Work out the finished part from the listing and answer in its coordinate system (mm). Face numbers are marked on the shaded views. A direction names the side the tool comes from. Give positions to 0.01 mm unless a question says otherwise; leave off trailing zeros. Order: outer loops, then holes, each group sorted by start corner. A loop starts at its lowest first (then second) coordinate and runs counter-clockwise, first axis right, second up. Notation, with made-up numbers: (-14, 17.5) - (30, 17.5) arc R31 ccw to (30, 45.5) - close; hole circle Ø8 at (30.5, 51.5). An arc over 180 degrees is marked (long way). Return JSON: item names as keys, results as strings. Group by question number.
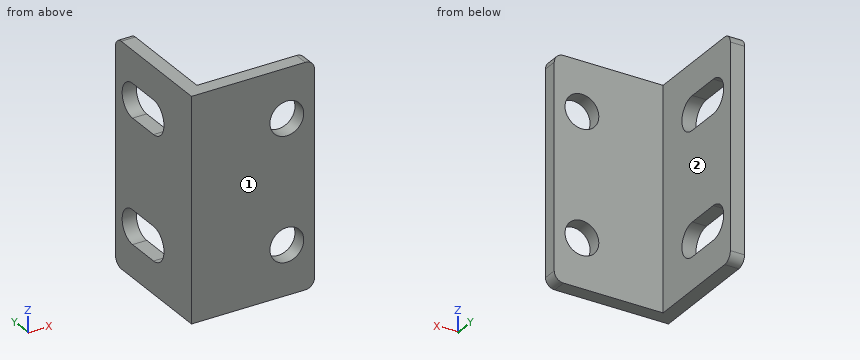
Autodesk Inventor part; units mm, degrees
ref_plane "to_cbm_1_1_XY" through (2.3, 15.5, -10) normal (1, 0, 0) x (0, 0, -1)
ref_plane "to_cbm_1_1_YZ" through (2.3, 15.5, -10) normal (0, 0, -1) x (0, 1, 0)
ref_plane "to_cbm_1_1_ZX" through (2.3, 15.5, -10) normal (0, 1, 0) x (1, 0, 0)
sketch "Sketch_2" plane through (0, 0, 0) normal (0, 1, 0) x (-1, 0, 0)
  line L0 (0, 18) -> (-18.5, 18)
  arc A0 (-18.5, 18) -> (-20, 16.5) centre (-18.5, 16.5) ccw
  line L1 (-20, 16.5) -> (-20, -16.5)
  arc A1 (-20, -16.5) -> (-18.5, -18) centre (-18.5, -16.5) ccw
  line L2 (-18.5, -18) -> (0, -18)
  line L3 (0, -18) -> (0, 18)
  circle A2 centre (-15.5, -10) radius 2.75
  circle A3 centre (-15.5, 10) radius 2.75
extrude "Extrusion1" add sketch "Sketch_2" along normal blind 2.3
sketch "Sketch_1" plane through (0, 0, 0) normal (1, 0, 0) x (0, 1, 0)
  line L0 (18.5, 18) -> (0, 18)
  line L1 (0, 18) -> (0, -18)
  line L2 (0, -18) -> (18.5, -18)
  arc A0 (18.5, -18) -> (20, -16.5) centre (18.5, -16.5) ccw
  line L3 (20, -16.5) -> (20, 16.5)
  arc A1 (20, 16.5) -> (18.5, 18) centre (18.5, 16.5) ccw
  line L4 (15.5, -7.25) -> (10, -7.25)
  arc A2 (10, -7.25) -> (10, -12.75) centre (10, -10) ccw
  line L5 (10, -12.75) -> (15.5, -12.75)
  arc A3 (15.5, -12.75) -> (15.5, -7.25) centre (15.5, -10) ccw
  line L6 (15.5, 12.75) -> (10, 12.75)
  arc A4 (10, 12.75) -> (10, 7.25) centre (10, 10) ccw
  line L7 (10, 7.25) -> (15.5, 7.25)
  arc A5 (15.5, 7.25) -> (15.5, 12.75) centre (15.5, 10) ccw
extrude "Extrusion2" add sketch "Sketch_1" along normal blind 2.3
ref_plane "to_cbm_1_1_XY" through (2.3, 15.5, -10) normal (1, 0, 0) x (0, 0, -1)
ref_plane "to_cbm_1_1_YZ" through (2.3, 15.5, -10) normal (0, 0, -1) x (0, 1, 0)
ref_plane "to_cbm_1_1_ZX" through (2.3, 15.5, -10) normal (0, 1, 0) x (1, 0, 0)
ref_plane "to_cbm_1_2_XY" through (2.3, 15.5, 10) normal (1, 0, 0) x (0, 0, -1)
ref_plane "to_cbm_1_2_YZ" through (2.3, 15.5, 10) normal (0, 0, -1) x (0, 1, 0)
ref_plane "to_cbm_1_2_ZX" through (2.3, 15.5, 10) normal (0, 1, 0) x (1, 0, 0)
ref_plane "to_cbm_2_1_XY" through (15.5, 2.3, 10) normal (0, 1, 0) x (1, 0, 0)
ref_plane "to_cbm_2_1_YZ" through (15.5, 2.3, 10) normal (1, 0, 0) x (0, 0, -1)
ref_plane "to_cbm_2_1_ZX" through (15.5, 2.3, 10) normal (0, 0, -1) x (0, 1, 0)
ref_plane "to_cbm_2_2_XY" through (15.5, 2.3, -10) normal (0, 1, 0) x (1, 0, 0)
ref_plane "to_cbm_2_2_YZ" through (15.5, 2.3, -10) normal (1, 0, 0) x (0, 0, -1)
ref_plane "to_cbm_2_2_ZX" through (15.5, 2.3, -10) normal (0, 0, -1) x (0, 1, 0)
ref_plane "to_hntp5_1_1_XY" through (-2, 15.5, -10) normal (-1, 0, 0) x (0, -1, 0)
ref_plane "to_hntp5_1_1_YZ" through (-2, 15.5, -10) normal (0, -1, 0) x (0, 0, 1)
ref_plane "to_hntp5_1_1_ZX" through (-2, 15.5, -10) normal (0, 0, 1) x (-1, 0, 0)
ref_plane "to_hntp5_1_2_XY" through (-2, 15.5, 10) normal (-1, 0, 0) x (0, -1, 0)
ref_plane "to_hntp5_1_2_YZ" through (-2, 15.5, 10) normal (0, -1, 0) x (0, 0, 1)
ref_plane "to_hntp5_1_2_ZX" through (-2, 15.5, 10) normal (0, 0, 1) x (-1, 0, 0)
ref_plane "to_hntp5_2_1_XY" through (15.5, -2, 10) normal (0, -1, 0) x (-1, 0, 0)
ref_plane "to_hntp5_2_1_YZ" through (15.5, -2, 10) normal (-1, 0, 0) x (0, 0, -1)
ref_plane "to_hntp5_2_1_ZX" through (15.5, -2, 10) normal (0, 0, -1) x (0, -1, 0)
ref_plane "to_hntp5_2_2_XY" through (15.5, -2, -10) normal (0, -1, 0) x (-1, 0, 0)
ref_plane "to_hntp5_2_2_YZ" through (15.5, -2, -10) normal (-1, 0, 0) x (0, 0, -1)
ref_plane "to_hntp5_2_2_ZX" through (15.5, -2, -10) normal (0, 0, -1) x (0, -1, 0)
properties part number "HPTBD5-SEP_b."
1. Each of these flat-tipped pins is pushed along its axis until it touches: pin 1 (2 mm diameter, centred on x = 9.5, z = -11.5, fed in from -Y); pin 2 (6.5 mm diameter, centred on x = 15.5, z = 10, fed in from +Y). Where does it stop, or does it pass through?
2. A tool of negligible diameter and unlimited length cuts with its end or side. For the marked faces 1 and 2, from which of +Z, -Z, +X, -X, +Y, -Y can it reach the whole face along a straight path? Write none if from no direction.
3. The part is cut by section B-B (y = 14.5). Give the vertices of the cut face in (x, z).
4. The part is cut by section D-D (z = -5). Give the vertices of the cut face in (x, y), and give its area (3 significant figures).
5. The part is cut by section A-A (z = 10). Give the vertices of the cut face in (x, y), and give its area (3 significant figures).
6. Consider probe 1 along Z at (x, y) = (15.5, 1.3); probe 2 along Z at (x, y) = (13, 2); probe 3 along X at (y, z) = (4.75, -1). Determine where each line is inside the solid, lowest interval first. Write a range as from..to.
Answers:
{
 "1": {"pin 1": "stops at y = 0", "pin 2": "stops at y = 2.3"},
 "2": {"face 1": "+Z, -Z, +X, -X, -Y", "face 2": "+Z, -Z, +X, +Y"},
 "3": {"outline": "(0, -18) - (2.3, -18) - (2.3, -12.75) - (0, -12.75) - close; (0, -7.25) - (2.3, -7.25) - (2.3, 7.25) - (0, 7.25) - close; (0, 12.75) - (2.3, 12.75) - (2.3, 18) - (0, 18) - close"},
 "4": {"outline": "(0, 0) - (20, 0) - (20, 2.3) - (2.3, 2.3) - (2.3, 20) - (0, 20) - close", "area": "86.7 mm^2"},
 "5": {"outline": "(0, 0) - (12.75, 0) - (12.75, 2.3) - (2.3, 2.3) - (2.3, 7.25) - (0, 7.25) - close; (0, 18.25) - (2.3, 18.25) - (2.3, 20) - (0, 20) - close; (18.25, 0) - (20, 0) - (20, 2.3) - (18.25, 2.3) - close", "area": "48.8 mm^2"},
 "6": {"probe 1": "z = -18..-12.75, -7.25..7.25, 12.75..18", "probe 2": "z = -18..-11.15, -8.85..8.85, 11.15..18", "probe 3": "x = 0..2.3"}
}
